Here's how the part is built. I have some questions about the finished solid (model axes, mm). Face numbers are marked on the shaded views. A direction names the side the tool comes from. Give positions to 0.01 mm unless a question says otherwise; leave off trailing zeros. Loops run counter-clockwise (first coordinate to the right, second up) from the corner with the lowest first, then second, coordinate; pieces in that order, holes last. Notation, with made-up numbers: M -10,47 L 18,47 A38 ccw 18,86 Z; hole C 27.25,81.25 d7. An arc over 180 degrees is marked long. Answer as CSV lines item,"result". Start each with the question number.
Item 1: I want a section at D-D on z = 4. List the corners of the cut face in (x, y) for me.
Item 2: Will these pins go through, and if not, where does the flat tip stop? P1, Ø6, axis at x = 18.5, z = 26.5, coming from the +Y side; P2, Ø5.5, axis at y = -20, z = 15, coming from the +X side; P3, Ø4, axis at y = -5.5, z = 15, coming from the +X side.
Item 3: For the marked faces 1 and 2, which set-ups out of +Z, -Z, +X, -X, +Y, -Y let a thin tool reach every point of the face, with its end or its side?
Item 4: I want a section at A-A on y = -5.5. List the corners of the cut face in (x, z) for me.
Item 5: If I drill on line 1 along X through (y, z) = (-33.7, 15); line 2 along Z through (x, y) = (-9, -20); line 3 along X through (y, z) = (-8.5, 18), over which ranges is the centre line in solid material (lowest first)? Write a range as from..to.
Item 6: I want a section at C-C on z = 15. List the corners of the cut face in (x, y) for me, plus the area to 3 significant figures.
Item 7: I want a section at B-B on x = 11. List the corners of the cut face in (y, z) for me, plus the area to 3 significant figures.
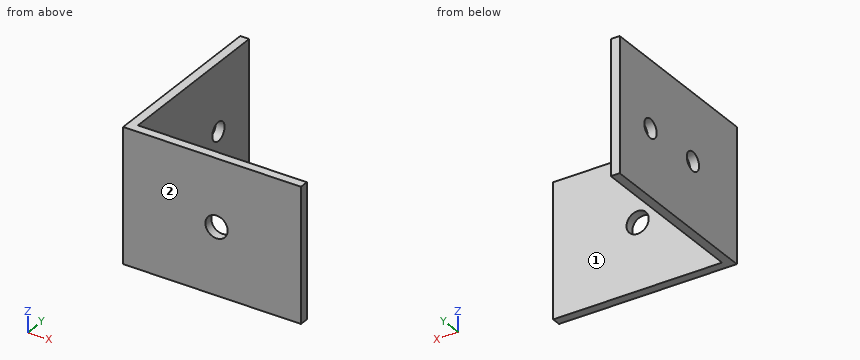
from build123d import *

# Parameters (mm, degrees)
BOSS_EXTRUDE1_DEPTH = 30
SKETCH2_R           = 2.1
CUT_EXTRUDE1_DEPTH  = 30
SKETCH3_R           = 2.5
CUT_EXTRUDE2_DEPTH  = 10


with BuildPart() as part:
    # Sketch1 → Boss-Extrude1 (new body)
    with BuildSketch(Plane.XY):
        Polygon((-8, 5), (-8, -33), (30, -33), (30, -35), (-10, -35), (-10, 5), align=None)
    extrude(amount=BOSS_EXTRUDE1_DEPTH)

    # Sketch2 → Cut-Extrude1 (cut)
    with BuildSketch(Plane(origin=(-8, 0, 0), x_dir=(0, 0, -1), z_dir=(1, 0, 0))):
        with Locations(Location((-15, -5.5, 0), (0, 0, 90))):
            Circle(SKETCH2_R)
        with Locations(Location((-15, -20, 0), (0, 0, 90))):
            Circle(SKETCH2_R)
    extrude(amount=-CUT_EXTRUDE1_DEPTH, mode=Mode.SUBTRACT)

    # Sketch3 → Cut-Extrude2 (cut)
    with BuildSketch(Plane(origin=(0, -33, 0), x_dir=(1, 0, 0), z_dir=(0, 1, 0))):
        with Locations(Location((11, -15, 0), (0, 0, 270))):
            Circle(SKETCH3_R)
    extrude(amount=-CUT_EXTRUDE2_DEPTH, mode=Mode.SUBTRACT)


solid = part.part
Result:
1,outline,"M -10,-35 L 30,-35 L 30,-33 L -8,-33 L -8,5 L -10,5 Z"
2,P1,"y = -33"
2,P2,"x = -8"
2,P3,"through"
3,face 1,"+Z, -Z, +X, +Y"
3,face 2,"+Z, -Z, +X, -X, -Y"
4,outline,"M -10,0 L -8,0 L -8,12.9 L -10,12.9 Z; M -10,17.1 L -8,17.1 L -8,30 L -10,30 Z"
5,line 1,"-10..8.5, 13.5..30"
5,line 2,"0..12.9, 17.1..30"
5,line 3,"-10..-8"
6,outline,"M -10,-35 L 8.5,-35 L 8.5,-33 L -8,-33 L -8,-22.1 L -10,-22.1 Z; M -10,-17.9 L -8,-17.9 L -8,-7.6 L -10,-7.6 Z; M -10,-3.4 L -8,-3.4 L -8,5 L -10,5 Z; M 13.5,-35 L 30,-35 L 30,-33 L 13.5,-33 Z"
6,area,"129 mm^2"
7,outline,"M -35,0 L -33,0 L -33,12.5 L -35,12.5 Z; M -35,17.5 L -33,17.5 L -33,30 L -35,30 Z"
7,area,"50.0 mm^2"
